Verification items for the finished model (mm, model axes). Face numbers are marked on the shaded views. A direction names the side the tool comes from. Give positions to 0.01 mm unless a question says otherwise; leave off trailing zeros. Loops run counter-clockwise (first coordinate to the right, second up) from the corner with the lowest first, then second, coordinate; pieces in that order, holes last. Notation, with made-up numbers: M 33,89 L 47,89 A19 ccw 47,118 Z; hole C 31.25,-0.75 d1. An arc over 180 degrees is marked long. Use CSV: the item, a comma, the result in double quotes.
from build123d import *

# Parameters (mm, degrees)
SKETCH1_R           = 30
SKETCH1_R_2         = 7
BOSS_EXTRUDE1_DEPTH = 10
FILLET1_R           = 20
FILLET2_R           = 10
CUT_EXTRUDE1_DEPTH  = 9.5


with BuildPart() as part:
    # Sketch1 → Boss-Extrude1 (new body, symmetric)
    with BuildSketch(Plane.XY):
        with BuildLine():
            Line((28.309347234, -25.349178669), (127.980959562, -8.974556643))
            ThreePointArc((127.980959562, -8.974556643), (155, 0), (127.980959562, 8.974556643))
            Line((127.980959562, 8.974556643), (28.309347234, 25.349178669))
            ThreePointArc((28.309347234, 25.349178669), (-38, 0), (28.309347234, -25.349178669))
        make_face()
        Circle(SKETCH1_R, mode=Mode.SUBTRACT)
        with Locations((140, 0)):
            Circle(SKETCH1_R_2, mode=Mode.SUBTRACT)
    extrude(amount=BOSS_EXTRUDE1_DEPTH, both=True)

    # Fillet1
    fillet1_edges = [part.edges().sort_by_distance(p)[0] for p in [
        (28.309347234, 25.349178669, 0),
        (28.309347234, -25.349178669, 0),
    ]]
    fillet(fillet1_edges, radius=FILLET1_R)

    # Fillet2
    fillet2_edges = [part.edges().sort_by_distance(p)[0] for p in [
        (127.980959562, 8.974556643, 0),
        (127.980959562, -8.974556643, 0),
    ]]
    fillet(fillet2_edges, radius=FILLET2_R)

    # Sketch2 → Cut-Extrude1 (cut)
    with BuildSketch(Plane.XY.offset(10)):
        with BuildLine():
            Line((38.638691874, 18.07848713), (121.848393563, 4.408321852))
            ThreePointArc((121.848393563, 4.408321852), (125.854189802, -0.497633455), (120.986555874, -4.549909473))
            Line((120.986555874, -4.549909473), (38.638691874, -18.07848713))
            ThreePointArc((38.638691874, -18.07848713), (34.002624892, -16.364178365), (33.10514216, -11.503468916))
            ThreePointArc((33.10514216, -11.503468916), (35.046829165, 0), (33.10514216, 11.503468916))
            ThreePointArc((33.10514216, 11.503468916), (34.002624892, 16.364178365), (38.638691874, 18.07848713))
        make_face()
    cut_extrude1 = extrude(amount=-CUT_EXTRUDE1_DEPTH, mode=Mode.SUBTRACT)

    # Mirror1: Cut-Extrude1 across plane
    add(cut_extrude1.mirror(Plane.XY), mode=Mode.SUBTRACT)


solid = part.part
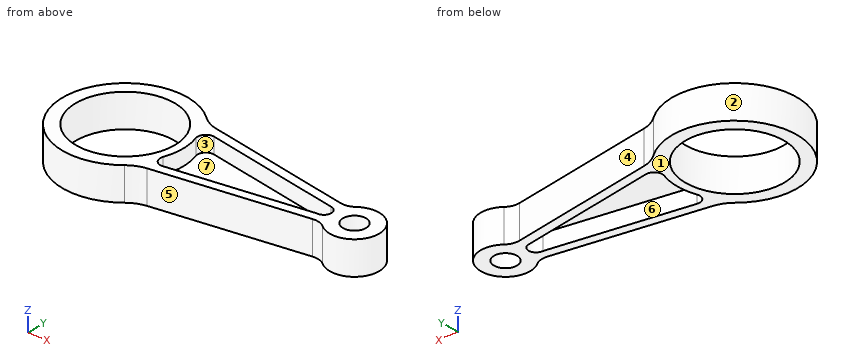
(1) Section check C-C on z = 5. Record the cut outline in (x, y).
Calculated:
outline,"M 24.7,-28.88 A20 cw 34.46,-24.34 L 122.95,-9.8 A10 cw 130.74,-11.8 A15 ccw long 130.74,11.8 A10 cw 122.95,9.8 L 34.46,24.34 A20 cw 24.7,28.88 A38 ccw long Z; hole C 0,0 d60; hole M 33.11,-11.5 A5 ccw 38.64,-18.08 L 120.99,-4.55 A4.5 ccw 121.85,4.41 L 38.64,18.08 A5 ccw 33.11,11.5 A35.05 cw Z; hole C 140,0 d14"
(2) Depth check by flat-ended pin: pin 1 Ø4 at (y, z) = (-17.5, 1) entering from -X; pin 2 Ø11 at (x, y) = (86.5, 4) entering from +Z; pin 3 Ø1.5 at (x, z) = (19, -5.5) entering from -Y. Enter the tip coordinate at first touch or a pass-through.
Calculated:
pin 1,"stops at x = -34.7"
pin 2,"stops at z = 0.5"
pin 3,"stops at y = -33.33"
(3) Tool access check on the marked faces 4, 5, 6 and 7. Record the directions out of +Z, -Z, +X, -X, +Y, -Y that give a thin tool (end or side, any length) a straight path to the whole face; none if there is none.
Calculated:
face 4,"+Z, -Z, +Y"
face 5,"+Z, -Z, -Y"
face 6,"-Z"
face 7,"+Z"
(4) Section check D-D on y = 0. Record the cut outline in (x, z).
Calculated:
outline,"M -38,-10 L -30,-10 L -30,10 L -38,10 Z; M 30,-10 L 35.05,-10 L 35.05,-0.5 L 125.87,-0.5 L 125.87,-10 L 133,-10 L 133,10 L 125.87,10 L 125.87,0.5 L 35.05,0.5 L 35.05,10 L 30,10 Z; M 147,-10 L 155,-10 L 155,10 L 147,10 Z"
(5) Scan lines: L1, parallel to Y at x = 140, z = -2; L2, parallel to Y at x = 0, z = 2; L3, parallel to X at y = -26.5, z = -4. Record each from-to range of solid material in increasing order. Write a range as from..to.
Calculated:
L1,"y = -15..-7, 7..15"
L2,"y = -38..-30, 30..38"
L3,"x = -27.24..-14.06, 14.06..28.16"
(6) Section check A-A on x = 140. Record the cut outline in (y, z), plus the area to 3 significant figures.
Calculated:
outline,"M -15,-10 L -7,-10 L -7,10 L -15,10 Z; M 7,-10 L 15,-10 L 15,10 L 7,10 Z"
area,"320 mm²"
(7) Mould release check, pull along X, two halves, no side actions. Record for the marked faces 1, 2 and 3: released by +X, released by -X, zero draft, split by the parting line, or undercut.
Calculated:
face 1,"zero draft"
face 2,"split by the parting line"
face 3,"undercut"
(8) Section check B-B on y = -26.5. Record the cut outline in (x, z).
Calculated:
outline,"M -27.24,-10 L -14.06,-10 L -14.06,10 L -27.24,10 Z; M 14.06,-10 L 28.16,-10 L 28.16,10 L 14.06,10 Z"
